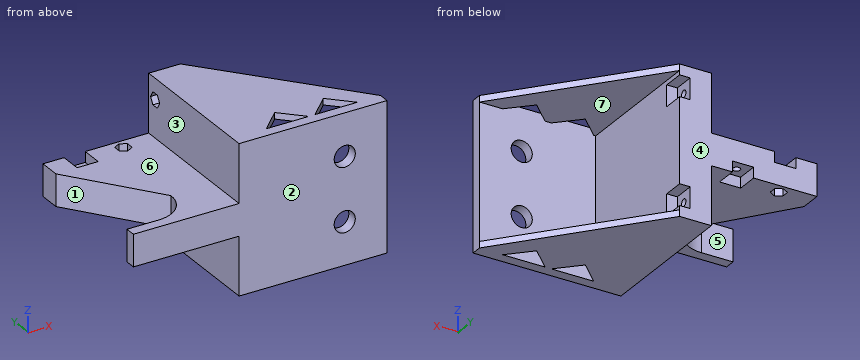
from build123d import *

# Parameters (mm, degrees)
SKETCH1_R           = 5
BOSS_EXTRUDE1_DEPTH = 5
BOSS_EXTRUDE2_DEPTH = 65
SKETCH3_W           = 15
SKETCH3_H           = 10
BOSS_EXTRUDE3_DEPTH = 30
CHAMFER2_SIZE2      = 40
CHAMFER2_SIZE       = 30
SKETCH4_W           = 10
SKETCH4_H           = 5
SKETCH4_W_2         = 5
SKETCH4_H_2         = 10
CUT_EXTRUDE1_DEPTH  = 10
CUT_EXTRUDE2_START  = -5
CUT_EXTRUDE2_DEPTH  = 10
SKETCH6_R           = 1.7
CUT_EXTRUDE3_DEPTH  = 10
SKETCH7_R           = 1.7
CUT_EXTRUDE4_DEPTH  = 10
CUT_EXTRUDE5_START  = -5
CUT_EXTRUDE5_DEPTH  = 10
SKETCH9_R           = 1.7
CUT_EXTRUDE6_DEPTH  = 10
CUT_EXTRUDE7_START  = -5
CUT_EXTRUDE7_DEPTH  = 10
FILLET2_R           = 15
BOSS_EXTRUDE4_DEPTH = 3


with BuildPart() as part:
    # Sketch1 → Boss-Extrude1 (new body)
    with BuildSketch(Plane(origin=(0, 0, 0), x_dir=(1, 0, 0), z_dir=(0, 1, 0))):
        Polygon((60, -35), (60, 35), (-10, 35), (-10, 7.5), (-60, 7.5), (-60, -7.5), (-10, -7.5), (-10, -35), align=None)
        with Locations(Location((40, 15, 0), (0, 0, 270))):
            Circle(SKETCH1_R, mode=Mode.SUBTRACT)
        with Locations(Location((40, -15, 0), (0, 0, 270))):
            Circle(SKETCH1_R, mode=Mode.SUBTRACT)
    extrude(amount=BOSS_EXTRUDE1_DEPTH)

    # Sketch2 → Boss-Extrude2 (add)
    with BuildSketch(Plane(origin=(0, 5, 0), x_dir=(1, 0, 0), z_dir=(0, 1, 0))):
        Polygon((-10, 35), (-10, 7.5), (-30, 7.5), (-30, -7.5), (-10, -7.5), (-10, -35), (5, -35), (5, 35), align=None)
    extrude(amount=BOSS_EXTRUDE2_DEPTH)

    # Sketch3 → Boss-Extrude3 (add)
    with BuildSketch(Plane.ZY.offset(30)):
        with Locations((0, 65)):
            Rectangle(SKETCH3_W, SKETCH3_H)
    extrude(amount=BOSS_EXTRUDE3_DEPTH)

    # Chamfer2
    chamfer2_edges = [part.edges().sort_by_distance(p)[0] for p in [
        (-30, 60, 0),
    ]]
    chamfer2_side = [part.faces().sort_by_distance(p)[0] for p in [
        (-30.6, 60, 0),
    ]]
    chamfer(chamfer2_edges, length=CHAMFER2_SIZE - 0.0001, length2=CHAMFER2_SIZE2 - 0.0001, reference=chamfer2_side[0])  # a hair under: the kernel refuses the full size

    # Sketch4 → Cut-Extrude1 (cut)
    with BuildSketch(Plane(origin=(0, 70, 0), x_dir=(1, 0, 0), z_dir=(0, 1, 0))):
        with Locations((-25, 5)):
            Rectangle(SKETCH4_W, SKETCH4_H)
        with Locations((-45, -5)):
            Rectangle(SKETCH4_W, SKETCH4_H)
        with Locations((2.5, 25)):
            Rectangle(SKETCH4_W_2, SKETCH4_H_2)
        with Locations((2.5, -25)):
            Rectangle(SKETCH4_W_2, SKETCH4_H_2)
    extrude(amount=-CUT_EXTRUDE1_DEPTH, mode=Mode.SUBTRACT)

    # Sketch5 → Cut-Extrude2 (cut)
    with BuildSketch(Plane(origin=(0, 0, 0), x_dir=(0, 0, -1), z_dir=(1, 0, 0)).offset(CUT_EXTRUDE2_START)):
        Polygon((-25, 61.5), (-21.968911087, 63.25), (-21.968911087, 66.75), (-25, 68.5), (-28.031088913, 66.75), (-28.031088913, 63.25), align=None)
    cut_extrude2 = extrude(amount=-CUT_EXTRUDE2_DEPTH, mode=Mode.SUBTRACT)

    # Sketch6 → Cut-Extrude3 (cut)
    with BuildSketch(Plane(origin=(0, 0, 0), x_dir=(0, 0, -1), z_dir=(1, 0, 0))):
        with Locations((-25, 65)):
            Circle(SKETCH6_R)
    cut_extrude3 = extrude(amount=-CUT_EXTRUDE3_DEPTH, mode=Mode.SUBTRACT)

    # Mirror1: Cut-Extrude2 across plane
    add(cut_extrude2.mirror(Plane.XY), mode=Mode.SUBTRACT)

    # Mirror2: Cut-Extrude3 across plane
    add(cut_extrude3.mirror(Plane.XY), mode=Mode.SUBTRACT)

    # Sketch7 → Cut-Extrude4 (cut)
    with BuildSketch(Plane.XY.offset(2.5)):
        with Locations((-45, 65)):
            Circle(SKETCH7_R)
    extrude(amount=-CUT_EXTRUDE4_DEPTH, mode=Mode.SUBTRACT)

    # Sketch8 → Cut-Extrude5 (cut)
    with BuildSketch(Plane.XY.offset(2.5).offset(CUT_EXTRUDE5_START)):
        Polygon((-45, 68.5), (-48.031088913, 66.75), (-48.031088913, 63.25), (-45, 61.5), (-41.968911087, 63.25), (-41.968911087, 66.75), align=None)
    extrude(amount=-CUT_EXTRUDE5_DEPTH, mode=Mode.SUBTRACT)

    # Sketch9 → Cut-Extrude6 (cut)
    with BuildSketch(Plane(origin=(0, 0, -2.5), x_dir=(-1, 0, 0), z_dir=(0, 0, -1))):
        with Locations((25, 65)):
            Circle(SKETCH9_R)
    extrude(amount=-CUT_EXTRUDE6_DEPTH, mode=Mode.SUBTRACT)

    # Sketch10 → Cut-Extrude7 (cut)
    with BuildSketch(Plane(origin=(0, 0, -2.5), x_dir=(-1, 0, 0), z_dir=(0, 0, -1)).offset(CUT_EXTRUDE7_START)):
        Polygon((25, 68.5), (21.968911087, 66.75), (21.968911087, 63.25), (25, 61.5), (28.031088913, 63.25), (28.031088913, 66.75), align=None)
    extrude(amount=-CUT_EXTRUDE7_DEPTH, mode=Mode.SUBTRACT)

    # Fillet2
    fillet2_edges = [part.edges().sort_by_distance(p)[0] for p in [
        (-30, 5, 0),
    ]]
    fillet(fillet2_edges, radius=FILLET2_R)

    # Sketch11 → Boss-Extrude4 (add)
    with BuildSketch(Plane(origin=(0, 0, -35), x_dir=(-1, 0, 0), z_dir=(0, 0, -1))):
        Polygon((-5, 70), (-60, 5), (-49, 5), (-39, 15), (-29, 5), (-26, 5), (-16, 15), (-6, 5), (-5, 5), align=None)
    boss_extrude4 = extrude(amount=-BOSS_EXTRUDE4_DEPTH)

    # Mirror3: Boss-Extrude4 across plane
    add(boss_extrude4.mirror(Plane.XY))


solid = part.part
Read the model definition and answer for the solid it produces. Units are mm, in the model's axes. Face numbers are marked on the shaded views. A direction names the side the tool comes from. Coordinates: 2 decimals unless noted, no trailing zeros. Loops run counter-clockwise (first coordinate to the right, second up) from the corner with the lowest first, then second, coordinate; pieces in that order, holes last.
Q1. Each of these flat-tipped pins is pushed along its axis until it touches: pin 1 Ø1.5 at (x, z) = (23, -25.5) entering from +Y; pin 2 Ø2 at (y, z) = (36, -18) entering from -X; pin 3 Ø5 at (y, z) = (13.5, -4) entering from -X; pin 4 Ø9 at (x, z) = (40, -15) entering from +Y. Where does it stop, or does it pass through?
Q2. The part is cut by section D-D on y = 31.5. Write down the section's boundary in (x, z).
Q3. The part is cut by section A-A on z = 15. Write down the section's boundary in (x, y).
Q4. Which of the six approach directions +Z, -Z, +X, -X, +Y, -Y give full straight-line access (tool end or side, diameter ignored) to the marked faces 5, 6 and 7?
Q5. The part is cut by section B-B on z = 1. Give the number of separate pieces and of enclosed holes in the cut face, and give its area (3 significant figures).
Q6. Consider probe 1 along X at (y, z) = (65, -0.6); probe 2 along Z at (x, y) = (-3, 65); probe 3 along X at (y, z) = (1, -15). Determine where each line is inside the solid, lowest interval first.
Q7. The mould has two halves that part along Y. Classify the marked faces 1, 2, 3 and 4: +Y half, -Y half, draft (parallel to the pull), parting line (faces both ways), or undercut.
Q8. The part is cut by section C-C on x = 21. Write down the section's boundary in (y, z), and give its area (3 significant figures).
Results below:
1. pin 1: stops at y = 5
1. pin 2: stops at x = -10
1. pin 3: stops at x = -33
1. pin 4: passes through
2. outline: (-38.62, -7.5) - (-10, -7.5) - (-10, -35) - (37.58, -35) - (37.58, -32) - (5, -32) - (5, 32) - (37.58, 32) - (37.58, 35) - (-10, 35) - (-10, 7.5) - (-38.62, 7.5) - close
3. outline: (-10, 0) - (35, 0) - (35, 5) - (5, 5) - (5, 70) - (-10, 70) - close; (45, 0) - (60, 0) - (60, 5) - (45, 5) - close
4. face 5: +Z, -Z, -X
4. face 6: +Z, -X, +Y, -Y
4. face 7: +X, +Y
5. separate pieces: 1
5. enclosed holes: 2
5. area: 3,810 mm2
6. probe 1: x = -60 to -46.7, -43.3 to -26.7, -23.3 to 5
6. probe 2: z = -35 to -26.7, -23.3 to 23.3, 26.7 to 35
6. probe 3: x = -10 to 35, 45 to 60
7. face 1: undercut
7. face 2: -Y half
7. face 3: draft
7. face 4: +Y half
8. outline: (0, -35) - (5, -35) - (5, 35) - (0, 35) - close; (10, -35) - (51.09, -35) - (51.09, -32) - (10, -32) - close; (10, 32) - (51.09, 32) - (51.09, 35) - (10, 35) - close
8. area: 597 mm2
